Can you work these out from the model? Positions are in its coordinate system, mm. A direction names the side the tool comes from. Coordinates: 2 decimals unless noted, no trailing zeros. Order: outer loops, then holes, each group sorted by start corner. A loop starts at its lowest first (then second) coordinate and runs counter-clockwise, first axis right, second up. Notation, with made-up numbers: (38, 11.25) -> (85, 11.25) arc R24 cw to (85, 48.25) -> close; hole circle Ø1 at (48.25, 53.25). An arc over 180 degrees is marked (long way). Return JSON: item names as keys, results as strings. Group by question number.
1) If we section it at C-C, the plane y = 2.5: State how many separate pieces and enclosed holes the cut face has, then the cut area to 3 significant figures.
2) For pin 1 (3 mm diameter, centred on x = 0, z = 31.5, fed in from +Y); pin 2 (1.5 mm diameter, centred on x = -28.5, y = 0.5, fed in from +Z); pin 3 (3 mm diameter, centred on y = -1.5, z = -3.5, fed in from -X), each with a flat end and sliding along its axis, tell me the tip position at first contact or that it passes through.
3) If we section it at B-B, the plane z = 0: Please give me the cut outline in (x, y).
4) If I drill on probe 1 along X at (y, z) = (2, 15.75); probe 2 along Z at (x, y) = (0.5, 3.25); probe 3 along X at (y, z) = (-0.5, 0), over which ranges is the centre line in solid material (lowest first)? Write a range as from..to.
5) If we section it at D-D, the plane z = -15.75: Please give me the cut outline in (x, y), then the cut area to 3 significant figures.
6) Thinking about a two-plate mould opening in X: for faces 1 (the cylindrical face through (-27.197, 1.912, 13.877)), 2 (the cylindrical face through (10.81, 0.06, 34.34)), 3 (the flat face through (-7, -4.119, -1)), which applies, +X half, -X half, draft (parallel to the pull), parting line (faces both ways), or undercut?
7) For faces 4 (the flat face through (-7, 4.131, -1)), 5 (the cylindrical face through (25.62, 1.91, 16.62)), which set-ups out of +Z, -Z, +X, -X, +Y, -Y let a thin tool reach every point of the face, with its end or its side?
8) If we section it at A-A, the plane x = 0: Please give me the cut outline in (y, z) (3 decimals).
from build123d import *

# Parameters (mm, degrees)
SKETCH_1_R               = 24
EXTRUDE_1_DEPTH          = 2.75
SKETCH_4_R               = 2.5
CUT_EXTRUDE_1_DEPTH      = 22
SKETCH_6_R               = 1.25
CUT_EXTRUDE_3_DEPTH      = 3
PATTERN_CIRCULAR_1_COUNT = 6
SCALE_1_SCALE            = 1.5


with BuildPart() as part:
    # 草图1 → 凸台-拉伸1 (new, symmetric)
    with BuildSketch(Plane(origin=(0, 0, 0), x_dir=(1, 0, 0), z_dir=(0, 1, 0))):
        with Locations(Location((0, 0, 0), (0, 0, 270))):
            Circle(SKETCH_1_R)
    extrude(amount=EXTRUDE_1_DEPTH, both=True)

    # 草图4 → 切除-拉伸1 (cut)
    with BuildSketch(Plane(origin=(0, 2.75, 0), x_dir=(1, 0, 0), z_dir=(0, 1, 0))):
        with Locations(Location((0, 0, 0), (0, 0, 270))):
            Circle(SKETCH_4_R)
    extrude(amount=-CUT_EXTRUDE_1_DEPTH, mode=Mode.SUBTRACT)

    # 草图6 → 切除-拉伸3 (cut)
    with BuildSketch(Plane(origin=(0, 2.75, 0), x_dir=(1, 0, 0), z_dir=(0, 1, 0))):
        with Locations(Location((0, 21, 0), (0, 0, 270))):
            Circle(SKETCH_6_R)
    cut_extrude_3 = extrude(amount=-CUT_EXTRUDE_3_DEPTH, mode=Mode.SUBTRACT)

    # 阵列(圆周)1: 切除-拉伸3 ×6 about axis
    pattern_circular_1_axis = Axis((0, 0, 0), (0, 1, 0))
    for i in range(1, PATTERN_CIRCULAR_1_COUNT):
        add(cut_extrude_3.rotate(pattern_circular_1_axis, i * 360 / PATTERN_CIRCULAR_1_COUNT), mode=Mode.SUBTRACT)


with BuildPart() as part_1:
    # 缩放比例1: scaled about (0, -0.011320641, 0)
    add(part.part.scale(SCALE_1_SCALE).moved(Location((0, 0.00566032, 0))))


solid = part_1.part
Result sheet:
{
 "1": {"separate pieces": "1", "enclosed holes": "7", "area": "3,960 mm2"},
 "2": {"pin 1": "stops at y = -0.37", "pin 2": "stops at z = 22.93", "pin 3": "stops at x = -35.94"},
 "3": {"outline": "(-36, -4.12) -> (-3.75, -4.12) -> (-3.75, 4.13) -> (-36, 4.13) -> close; (3.75, -4.12) -> (36, -4.12) -> (36, 4.13) -> (3.75, 4.13) -> close"},
 "4": {"probe 1": "x = -32.37..-29.15, -25.4..25.4, 29.15..32.37", "probe 2": "z = -36..-33.31, -29.69..-3.72, 3.72..29.69, 33.31..36", "probe 3": "x = -36..-3.75, 3.75..36"},
 "5": {"outline": "(-32.37, -4.12) -> (32.37, -4.12) -> (32.37, 4.13) -> (29.15, 4.13) -> (29.15, -0.37) -> (25.4, -0.37) -> (25.4, 4.13) -> (-25.4, 4.13) -> (-25.4, -0.37) -> (-29.15, -0.37) -> (-29.15, 4.13) -> (-32.37, 4.13) -> close", "area": "500 mm2"},
 "6": {"face 1": "undercut", "face 2": "parting line", "face 3": "draft"},
 "7": {"face 4": "+Z, -Z, +X, -X, +Y", "face 5": "+Y"},
 "8": {"outline": "(-4.119, -36) -> (4.131, -36) -> (4.131, -33.375) -> (-0.369, -33.375) -> (-0.369, -29.625) -> (4.131, -29.625) -> (4.131, -3.75) -> (-4.119, -3.75) -> close; (-4.119, 3.75) -> (4.131, 3.75) -> (4.131, 29.625) -> (-0.369, 29.625) -> (-0.369, 33.375) -> (4.131, 33.375) -> (4.131, 36) -> (-4.119, 36) -> close"}
}
